The model under review builds one solid part; all positions refer to its coordinate system, in mm. A direction names the side the tool comes from. Give positions to 0.01 mm unless a question says otherwise; leave off trailing zeros. Write each loop counter-clockwise with the first axis right and the second up, starting at its lowest first coordinate (ties: lowest second). Pieces come first, ordered by that corner, then holes. Notation, with made-up numbers: M 86,89 L 109,89 A20 ccw 109,111 Z; hole C 7,-25.5 d2. An arc over 180 degrees is marked long. Write item = value, one per line. Start each with the question number.
Autodesk Inventor part; units mm, degrees
ref_plane "YZ Plane" through (0, 0, 0) normal (1, 0, 0) x (0, 1, 0)
ref_plane "XZ Plane" through (0, 0, 0) normal (0, 1, 0) x (-1, 0, 0)
ref_plane "XY Plane" through (0, 0, 0) normal (0, 0, 1) x (1, 0, 0)
sketch "Sketch1" plane through (0, 0, 0) normal (0, 1, 0) x (-1, 0, 0)
  circle A0 centre (0, 0) radius 2.4498
  circle A1 centre (0, 0) radius 3.2766
  circle A2 centre (0, 0) radius 3.8989
  dimension "d0" = 4.8997
  dimension "d1" = 6.5532
  dimension "d2" = 7.7978
extrude "Extrusion1" add sketch "Sketch1" along normal blind 1.9837 contours A0
sketch "Sketch2" plane through (0, 0, 0) normal (0, -1, 0) x (1, 0, 0)
  circle A0 centre (0, 0) radius 3.9243
  dimension "d5" = 7.8486
extrude "Extrusion2" add sketch "Sketch2" along normal blind 1.0211
sketch "Sketch3" plane through (0, -1.0211, 0) normal (0, -1, 0) x (1, 0, 0)
  circle A0 centre (0, 0) radius 3.2766
  circle A1 centre (0, 0) radius 2.4511
  dimension "d8" = 6.5532
  dimension "d9" = 4.9022
extrude "Extrusion3" add sketch "Sketch3" along normal blind 2.225
properties part number "1x1 circular almost looks like peg peg"
Item 1: The part is to be moulded in two halves that separate along Z. For faces 1 (the flat face through (2, 0, 2)), 2 (the flat face through (0, -1.021, 0)), 3 (the cylindrical face through (3.743, -0.503, -1.179)), say which applies: released by +Z, released by -Z, zero draft, split by the parting line, or undercut.
Item 2: We need section A-A, the plane x = 0. Write out the cut boundary in (y, z).
Item 3: We need section C-C, the plane y = -1.35. Write out the cut boundary in (x, z).
Item 4: Clearance check with flat-ended pins moving along their axes: P1, Ø1.5, axis at x = -0.5, z = 0.5, coming from the -Y side; P2, Ø1, axis at x = 1, y = 1, coming from the -Z side. State where each tip first meets the part, or that it passes through.
Item 5: We need section D-D, the plane y = 0.7. Write out the cut boundary in (x, z).
Item 6: For faces 4 (the flat face through (0, 1.984, 0)), 5 (the cylindrical face through (2.338, -2.118, -0.736)), 6 (the cylindrical face through (-2.337, 0.978, -0.736)), list the 3-axis set-ups (+Z, -Z, +X, -X, +Y, -Y) from which the entire face can be reached by the end or side of a thin tool; tool diameter is ignored.
Item 7: We need section B-B, the plane z = 0. Write out the cut boundary in (x, y).
Item 8: To check wall thickness, follow probe 1 along Z at (x, y) = (0, -2.7); probe 2 along Y at (x, z) = (0.5, -1.5); probe 3 along Y at (x, z) = (2.25, -3). State the ranges of each line that lie inside material, in increasing order. Write a range as [from, to].
Worked out:
q1.face_1 = zero draft
q1.face_2 = undercut
q1.face_3 = split by the parting line
q2.outline = M -3.25,-3.28 L -1.02,-3.28 L -1.02,-3.92 L 0,-3.92 L 0,-2.45 L 1.98,-2.45 L 1.98,2.45 L 0,2.45 L 0,3.92 L -1.02,3.92 L -1.02,3.28 L -3.25,3.28 L -3.25,2.45 L -1.02,2.45 L -1.02,-2.45 L -3.25,-2.45 Z
q3.outline = C 0,0 d6.55; hole C 0,0 d4.9
q4.P1 = -1.02
q4.P2 = -2.4
q5.outline = C 0,0 d4.9
q6.face_4 = +Z, -Z, +X, -X, +Y
q6.face_5 = -Y
q6.face_6 = +Y
q7.outline = M -3.92,-1.02 L -3.28,-1.02 L -3.28,-3.25 L -2.45,-3.25 L -2.45,-1.02 L 2.45,-1.02 L 2.45,-3.25 L 3.28,-3.25 L 3.28,-1.02 L 3.92,-1.02 L 3.92,0 L 2.45,0 L 2.45,1.98 L -2.45,1.98 L -2.45,0 L -3.92,0 Z
q8.probe_1 = [-3.28, -2.45], [2.45, 3.28]
q8.probe_2 = [-1.02, 1.98]
q8.probe_3 = [-1.02, 0]
